```python
from build123d import *

# Parameters (mm, degrees)
F0_W       = 330
F0_H       = 330
F0_R       = 1.5
F0_R_2     = 2.6
F1_DEPTH   = 3
F2_SIZE2   = 1.849213
F2_SIZE    = 2.99999
F3_SIZE2   = 1.849213
F3_SIZE    = 2.99999
F3_2_SIZE2 = 1.849213
F3_2_SIZE  = 2.99999
F3_3_SIZE2 = 1.849213
F3_3_SIZE  = 2.99999
F3_4_SIZE2 = 1.849213
F3_4_SIZE  = 2.99999
F3_5_SIZE2 = 1.849213
F3_5_SIZE  = 2.99999
F3_6_SIZE2 = 1.849213
F3_6_SIZE  = 2.99999
F3_7_SIZE2 = 1.849213
F3_7_SIZE  = 2.99999
F3_8_SIZE2 = 1.849213
F3_8_SIZE  = 2.99999
F3_9_SIZE2 = 1.849213
F3_9_SIZE  = 2.99999


# Not quite as in the source:
# - a fillet or chamfer is up to 0.001 mm smaller than in the source, because OpenCascade refuses the exact size


with BuildPart() as f1:
    # F0 (on Top) → F1 (new body)
    with BuildSketch(Plane.XY):
        Rectangle(F0_W, F0_H)
        with Locations((-160.5, -160.5)):
            Circle(F0_R, mode=Mode.SUBTRACT)
        with Locations((-132.5, -95)):
            Circle(F0_R_2, mode=Mode.SUBTRACT)
        with Locations((-142.5, -75)):
            Circle(F0_R_2, mode=Mode.SUBTRACT)
        with Locations((13, -161)):
            Circle(F0_R, mode=Mode.SUBTRACT)
        with Locations((0, -95)):
            Circle(F0_R_2, mode=Mode.SUBTRACT)
        with Locations((160.5, -160.5)):
            Circle(F0_R, mode=Mode.SUBTRACT)
        with Locations((132.5, -95)):
            Circle(F0_R_2, mode=Mode.SUBTRACT)
        with Locations((142.5, -75)):
            Circle(F0_R_2, mode=Mode.SUBTRACT)
        with Locations((162, -3)):
            Circle(F0_R, mode=Mode.SUBTRACT)
        with Locations((-162, 2)):
            Circle(F0_R, mode=Mode.SUBTRACT)
        with Locations((-142.5, 75)):
            Circle(F0_R_2, mode=Mode.SUBTRACT)
        with Locations((-132.5, 95)):
            Circle(F0_R_2, mode=Mode.SUBTRACT)
        with Locations((-160.5, 160.5)):
            Circle(F0_R, mode=Mode.SUBTRACT)
        with Locations((142.5, 75)):
            Circle(F0_R_2, mode=Mode.SUBTRACT)
        with Locations((0, 95)):
            Circle(F0_R_2, mode=Mode.SUBTRACT)
        with Locations((24, 160.5)):
            Circle(F0_R, mode=Mode.SUBTRACT)
        with Locations((132.5, 95)):
            Circle(F0_R_2, mode=Mode.SUBTRACT)
        with Locations((160.5, 160.5)):
            Circle(F0_R, mode=Mode.SUBTRACT)
    extrude(amount=F1_DEPTH)

    # F2 (size 3 and 1.8492230955 in the source; OpenCascade refuses exactly that, so slightly less here)
    f2_edges = [f1.edges().sort_by_distance(p)[0] for p in [
        (-135.1, 95, 3),
    ]]
    f2_side = f1.faces().sort_by_distance((-135.1, 95, 1.5))[0]
    chamfer(f2_edges, length=F2_SIZE, length2=F2_SIZE2, reference=f2_side)

    # F3 (size 3 and 1.8492230955 in the source; OpenCascade refuses exactly that, so slightly less here)
    f3_edges = [f1.edges().sort_by_distance(p)[0] for p in [
        (-145.1, 75, 3),
    ]]
    f3_side = f1.faces().sort_by_distance((-145.1, 75, 1.5))[0]
    chamfer(f3_edges, length=F3_SIZE, length2=F3_SIZE2, reference=f3_side)

    # F3#2 (size 3 and 1.8492230955 in the source; OpenCascade refuses exactly that, so slightly less here)
    f3_2_edges = [f1.edges().sort_by_distance(p)[0] for p in [
        (-2.6, 95, 3),
    ]]
    f3_2_side = f1.faces().sort_by_distance((-2.6, 95, 1.5))[0]
    chamfer(f3_2_edges, length=F3_2_SIZE, length2=F3_2_SIZE2, reference=f3_2_side)

    # F3#3 (size 3 and 1.8492230955 in the source; OpenCascade refuses exactly that, so slightly less here)
    f3_3_edges = [f1.edges().sort_by_distance(p)[0] for p in [
        (129.9, 95, 3),
    ]]
    f3_3_side = f1.faces().sort_by_distance((129.9, 95, 1.5))[0]
    chamfer(f3_3_edges, length=F3_3_SIZE, length2=F3_3_SIZE2, reference=f3_3_side)

    # F3#4 (size 3 and 1.8492230955 in the source; OpenCascade refuses exactly that, so slightly less here)
    f3_4_edges = [f1.edges().sort_by_distance(p)[0] for p in [
        (139.9, 75, 3),
    ]]
    f3_4_side = f1.faces().sort_by_distance((139.9, 75, 1.5))[0]
    chamfer(f3_4_edges, length=F3_4_SIZE, length2=F3_4_SIZE2, reference=f3_4_side)

    # F3#5 (size 3 and 1.8492230955 in the source; OpenCascade refuses exactly that, so slightly less here)
    f3_5_edges = [f1.edges().sort_by_distance(p)[0] for p in [
        (139.9, -75, 3),
    ]]
    f3_5_side = f1.faces().sort_by_distance((139.9, -75, 1.5))[0]
    chamfer(f3_5_edges, length=F3_5_SIZE, length2=F3_5_SIZE2, reference=f3_5_side)

    # F3#6 (size 3 and 1.8492230955 in the source; OpenCascade refuses exactly that, so slightly less here)
    f3_6_edges = [f1.edges().sort_by_distance(p)[0] for p in [
        (129.9, -95, 3),
    ]]
    f3_6_side = f1.faces().sort_by_distance((129.9, -95, 1.5))[0]
    chamfer(f3_6_edges, length=F3_6_SIZE, length2=F3_6_SIZE2, reference=f3_6_side)

    # F3#7 (size 3 and 1.8492230955 in the source; OpenCascade refuses exactly that, so slightly less here)
    f3_7_edges = [f1.edges().sort_by_distance(p)[0] for p in [
        (-2.6, -95, 3),
    ]]
    f3_7_side = f1.faces().sort_by_distance((-2.6, -95, 1.5))[0]
    chamfer(f3_7_edges, length=F3_7_SIZE, length2=F3_7_SIZE2, reference=f3_7_side)

    # F3#8 (size 3 and 1.8492230955 in the source; OpenCascade refuses exactly that, so slightly less here)
    f3_8_edges = [f1.edges().sort_by_distance(p)[0] for p in [
        (-135.1, -95, 3),
    ]]
    f3_8_side = f1.faces().sort_by_distance((-135.1, -95, 1.5))[0]
    chamfer(f3_8_edges, length=F3_8_SIZE, length2=F3_8_SIZE2, reference=f3_8_side)

    # F3#9 (size 3 and 1.8492230955 in the source; OpenCascade refuses exactly that, so slightly less here)
    f3_9_edges = [f1.edges().sort_by_distance(p)[0] for p in [
        (-145.1, -75, 3),
    ]]
    f3_9_side = f1.faces().sort_by_distance((-145.1, -75, 1.5))[0]
    chamfer(f3_9_edges, length=F3_9_SIZE, length2=F3_9_SIZE2, reference=f3_9_side)


solid = f1.part
```
The listing builds one solid part. Answer for the finished solid, in the listing's coordinates (mm). Give positions to 0.01 mm unless a question says otherwise; leave off trailing zeros. Answer as CSV lines item,"result". Start each with the question number.
Q1. Determine the mould class of faces 1 (the conical face through (-142.854, 77.693, 0.188)), 2 (the conical face through (-0.59, -97.65, 0.19)), 3 (the flat face through (-2, 2, 3)) for opening direction X: pulls with the +X half, pulls with the -X half, needs draft (parallel to the pull), parting line crosses it, or undercut.
Q2. Given pin 1 (7 mm diameter, centred on x = -142.5, y = -75, fed in from +Z), flat-ended and moving along its own axis, determine where the tip first touches the part or whether it passes through.
Q3. Find the intervals of material crossed by L1, parallel to X at y = 160.5, z = 1.65; L2, parallel to X at y = -160.5, z = 0.8; L3, parallel to Y at x = -140, z = 2.9, in increasing order.
Results found:
1,face 1,"undercut"
1,face 2,"undercut"
1,face 3,"needs draft"
2,pin 1,"z = 1.46"
3,L1,"-165 to -162, -159 to 22.5, 25.5 to 159, 162 to 165"
3,L2,"-165 to -162, -159 to 11.59, 14.41 to 159, 162 to 165"
3,L3,"-165 to -78.61, -71.39 to 71.39, 78.61 to 165"
